For this review, take the finished solid that the model builds, in its own axes (mm). Face numbers are marked on the shaded views. Give positions to 0.01 mm unless a question says otherwise; leave off trailing zeros. Write each loop counter-clockwise with the first axis right and the second up, starting at its lowest first coordinate (ties: lowest second). Pieces come first, ordered by that corner, then holes.
Q1. We need section C-C (z = 14). Write out the cut boundary in (x, y).
Q2. We need section A-A (y = 19). Write out the cut boundary in (x, z).
Q3. We need section D-D (y = 7.5). Write out the cut boundary in (x, z).
Q4. Mouldability with a two-part tool opening along X and no side actions: class the marked faces 1, 2 and 3 as released by +X, released by -X, zero draft, split by the parting line, or undercut.
Q5. We need section B-B (x = 0). Write out the cut boundary in (y, z), then the cut area to 3 significant figures.
Q6. For line 1 (Y direction, x = 0, z = 19.25); line 2 (Y direction, x = 16, z = 13); line 3 (X direction, y = 0.5, z = 18.75), list the stretches that pass through material, from the lowest coordinate up.
Q7. Insertion check: P1, Ø3, axis at x = -17, y = 8.5, coming from the +Z side; P2, Ø2.5, axis at x = -5, z = 14, coming from the -Y side; P3, Ø1.5, axis at x = 18, z = 12.5, coming from the -Y side. Each pin has a flat end and moves straight along its axis. Give the tip position at first contact, or say it passes through.
Autodesk Inventor part; units mm, degrees
ref_plane "YZ Plane" through (0, 0, 0) normal (1, 0, 0) x (0, 1, 0)
ref_plane "XZ Plane" through (0, 0, 0) normal (0, 1, 0) x (-1, 0, 0)
ref_plane "XY Plane" through (0, 0, 0) normal (0, 0, 1) x (1, 0, 0)
sketch "Szkic1" plane through (0, 0, 0) normal (0, 0, 1) x (1, 0, 0)
  line L0 (-30, -30) -> (30, -30)
  line L1 (30, -30) -> (30, 30)
  line L2 (30, 30) -> (-30, 30)
  line L3 (-30, 30) -> (-30, -30)
  line L4 (-30, -30) -> (30, 30) construction
  line L5 (30, -30) -> (-30, 30) construction
  point P0 (0, 0)
  dimension "d0" = 60
  dimension "d1" = 60
extrude "Wyciągnięcie proste1" add sketch "Szkic1" along normal blind 35
sketch "Szkic2" plane through (0, 0, 35) normal (0, 0, 1) x (1, 0, 0)
  circle A0 centre (0, 0) radius 25
  dimension "d4" = 50
extrude "Wyciągnięcie proste2" cut sketch "Szkic2" against normal blind 12
sketch "Szkic3" plane through (0, 0, 23) normal (0, 0, 1) x (1, 0, 0)
  circle A0 centre (0, 0) radius 14
  dimension "d7" = 28
extrude "Wyciągnięcie proste3" cut sketch "Szkic3" against normal up to next
sketch "Szkic4" plane through (0, 0, 23) normal (0, 0, 1) x (1, 0, 0)
  circle A0 centre (0, 0) radius 19
  circle A1 centre (0, 19) radius 3
  circle A2 centre (-16.4545, 9.5) radius 3
  circle A3 centre (-16.4545, -9.5) radius 3
  circle A4 centre (0, -19) radius 3
  circle A5 centre (16.4545, -9.5) radius 3
  circle A6 centre (16.4545, 9.5) radius 3
  dimension "d10" = 38
  dimension "d11" = 6
  dimension "d14" = 360
sketch "Szkic13" plane through (0, 0, 35) normal (0, 0, 1) x (1, 0, 0)
  circle A0 centre (0, 0) radius 25
  line L0 (-30, -30) -> (30, -30)
  line L1 (30, -30) -> (30, 30)
  line L2 (30, 30) -> (-30, 30)
  line L3 (-30, 30) -> (-30, -30)
extrude "Wyciągnięcie proste10" cut sketch "Szkic13" against normal up to surface (12 mm away)
extrude "Wyciągnięcie proste11" cut sketch "Szkic4" against normal blind 15 contours A6 A0 | A0 A6 | A5 A0 | A0 A5 | A1 A0 | A0 A1 | A4 A0 | A0 A4 | A2 A0 | A0 A2 | A3 A0 | A0 A3
thread "Gwint7"
thread "Gwint8"
thread "Gwint9"
thread "Gwint10"
thread "Gwint11"
thread "Gwint12"
sketch "Szkic14" plane through (0, 0, 0) normal (0, 0, -1) x (-1, 0, 0)
  circle A0 centre (0, 0) radius 14
  line L0 (30, -30) -> (-30, -30)
  line L1 (30, 30) -> (30, -30)
  line L2 (-30, 30) -> (30, 30)
  line L3 (-30, -30) -> (-30, 30)
extrude "Wyciągnięcie proste12" cut sketch "Szkic14" against normal blind 3
sketch "Szkic15" plane through (-30, -30, 23) normal (0, -1, 0) x (1, 0, 0)
  line L0 (0, -20) -> (60, -20)
  line L1 (60, -20) -> (60, 0)
  line L2 (60, 0) -> (0, 0)
  line L3 (0, -20) -> (0, 0)
  line L4 (0, 0) -> (60, 0)
  line L5 (0, 0) -> (0, -10)
  line L6 (0, -10) -> (60, -10)
  line L7 (60, -20) -> (60, 0)
  line L8 (0, -10) -> (12, -10)
  line L9 (12, -10) -> (24, -10)
  line L10 (24, -10) -> (36, -10)
  line L11 (36, -10) -> (48, -10)
  circle A0 centre (12, -10) radius 2.5
  circle A1 centre (24, -10) radius 2.5
  circle A2 centre (36, -10) radius 2.5
  circle A3 centre (48, -10) radius 2.5
  point P0 (30, -23)
  dimension "d79" = 10
  dimension "d80" = 12
  dimension "d81" = 12
  dimension "d82" = 12
  dimension "d83" = 12
  dimension "d84" = 5
  dimension "d85" = 5
  dimension "d86" = 5
  dimension "d87" = 5
extrude "Wyciągnięcie proste13" cut sketch "Szkic15" against normal blind 8 contours A0 L6 | L6 A0 | A3 L6 | L6 A3 | A1 L6 | L6 A1 | A2 L6 | L6 A2
thread "Gwint13"
thread "Gwint14"
thread "Gwint15"
thread "Gwint16"
properties part number "Obudowa nakrętki trapezowej fi 16"
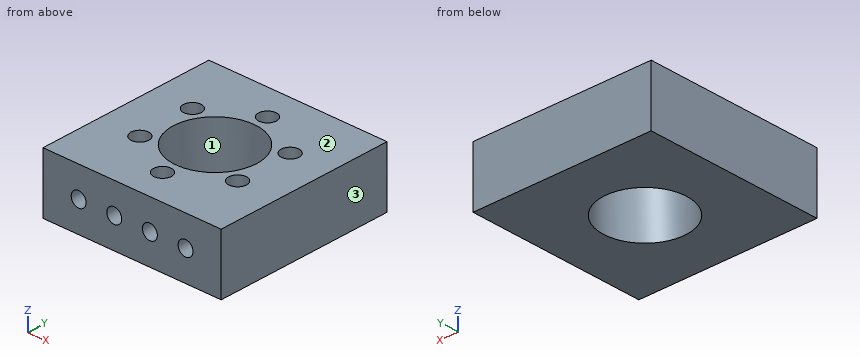
Computed:
1. outline: (-30, -30) - (-20.29, -30) - (-20.29, -22) - (-15.71, -22) - (-15.71, -30) - (-8.29, -30) - (-8.29, -22) - (-3.71, -22) - (-3.71, -30) - (3.71, -30) - (3.71, -22) - (8.29, -22) - (8.29, -30) - (15.71, -30) - (15.71, -22) - (20.29, -22) - (20.29, -30) - (30, -30) - (30, 30) - (-30, 30) - close; hole circle Ø6 at (-16.45, -9.5); hole circle Ø6 at (-16.45, 9.5); hole circle Ø28 at (0, 0); hole circle Ø6 at (0, -19); hole circle Ø6 at (0, 19); hole circle Ø6 at (16.45, -9.5); hole circle Ø6 at (16.45, 9.5)
2. outline: (-30, 3) - (30, 3) - (30, 23) - (3, 23) - (3, 8) - (-3, 8) - (-3, 23) - (-30, 23) - close
3. outline: (-30, 3) - (-11.82, 3) - (-11.82, 23) - (-14.22, 23) - (-14.22, 8) - (-18.69, 8) - (-18.69, 23) - (-30, 23) - close; (11.82, 3) - (30, 3) - (30, 23) - (18.69, 23) - (18.69, 8) - (14.22, 8) - (14.22, 23) - (11.82, 23) - close
4. face 1: undercut
4. face 2: zero draft
4. face 3: released by +X
5. outline: (-30, 3) - (-14, 3) - (-14, 23) - (-16, 23) - (-16, 8) - (-22, 8) - (-22, 23) - (-30, 23) - close; (14, 3) - (30, 3) - (30, 23) - (22, 23) - (22, 8) - (16, 8) - (16, 23) - (14, 23) - close
5. area: 460 mm2
6. line 1: y = -30 to -22, -16 to -14, 14 to 16, 22 to 30
6. line 2: y = -22 to -12.47, -6.53 to 6.53, 12.47 to 30
6. line 3: x = -30 to -13.99, 13.99 to 30
7. P1: stops at z = 8
7. P2: stops at y = -30
7. P3: stops at y = -22
